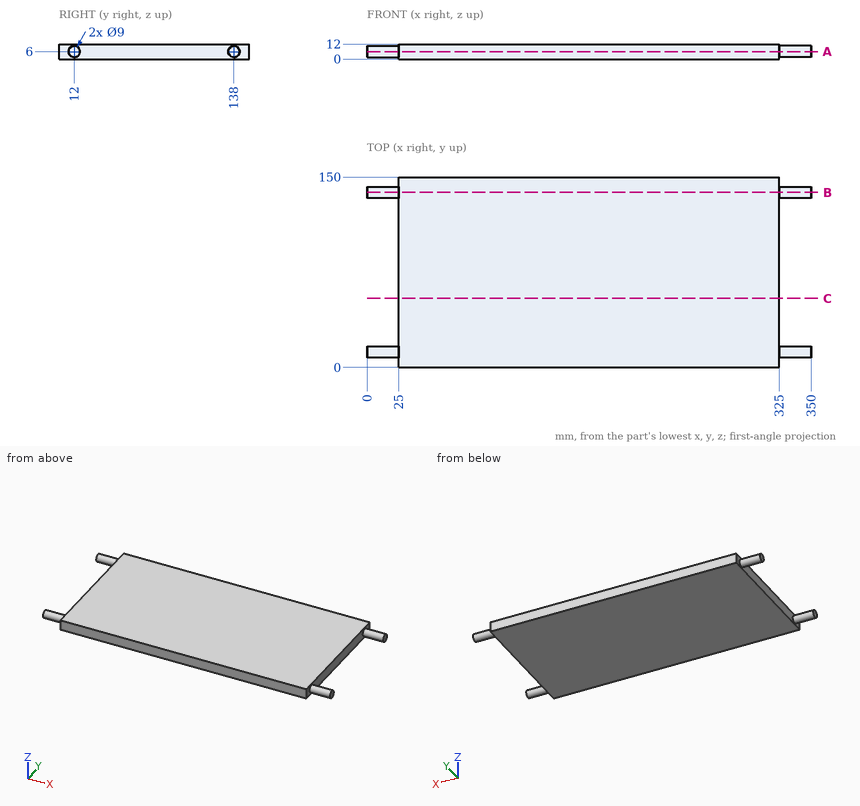
Geometry: see drawing. Coordinates: mm, zero at the bounding-box minimum. Coordinates: 2 decimals unless noted, no trailing zeros. Write each loop counter-clockwise with the first axis right and the second up, starting at its lowest first coordinate (ties: lowest second). Pieces come first, ordered by that corner, then holes. Notation, with made-up numbers: M 12,87 L 56,87 A24 cw 56,120 Z; hole C 15.5,-2.5 d4. An arc over 180 degrees is marked long. Use CSV: the item, a comma, the result in double quotes. Start each with the question number.
1. Cut plane C-C on y = 54.5. Return the cut outline in (x, z), plus the area to 3 significant figures.
2. Ray query, probe 1 along X at (y, z) = (128.5, 2). Return the intervals inside material, ascending.
3. First-contact query: P1, Ø2, axis at y = 51, z = 2, coming from the -X side. Flat tip, straight axial feed; report the tip coordinate or a pass-through.
4. Cut plane A-A on z = 6. Return the cut outline in (x, y), plus the area to 3 significant figures.
5. Cut plane B-B on y = 138. Return the cut outline in (x, z), plus the area to 3 significant figures.
Entries:
1,outline,"M 25,0 L 325,0 L 325,12 L 25,12 Z"
1,area,"3,600 mm²"
2,probe 1,"25 to 325"
3,P1,"x = 25"
4,outline,"M 0,7.5 L 25,7.5 L 25,0 L 325,0 L 325,7.5 L 350,7.5 L 350,16.5 L 325,16.5 L 325,133.5 L 350,133.5 L 350,142.5 L 325,142.5 L 325,150 L 25,150 L 25,142.5 L 0,142.5 L 0,133.5 L 25,133.5 L 25,16.5 L 0,16.5 Z"
4,area,"45,900 mm²"
5,outline,"M 0,1.5 L 25,1.5 L 25,0 L 325,0 L 325,1.5 L 350,1.5 L 350,10.5 L 325,10.5 L 325,12 L 25,12 L 25,10.5 L 0,10.5 Z"
5,area,"4,050 mm²"
